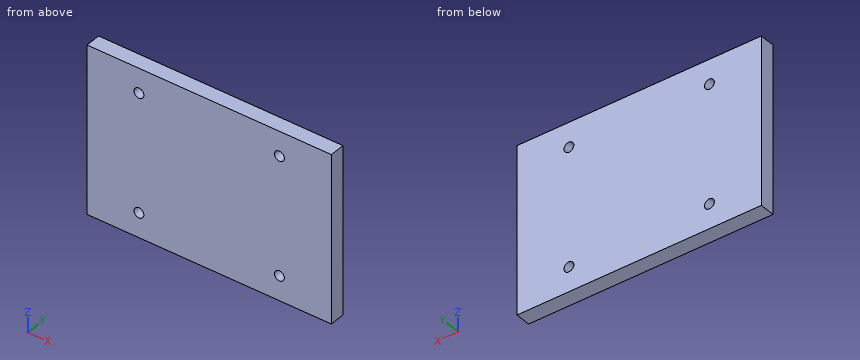
Autodesk Inventor part; units mm, degrees
ref_plane "YZ Plane" through (0, 0, 0) normal (1, 0, 0) x (0, 1, 0)
ref_plane "XZ Plane" through (0, 0, 0) normal (0, 1, 0) x (-1, 0, 0)
ref_plane "XY Plane" through (0, 0, 0) normal (0, 0, 1) x (1, 0, 0)
sketch "Boceto1" plane through (0, 0, 0) normal (0, 1, 0) x (-1, 0, 0)
  line L0 (0, 0) -> (-80, 0)
  line L1 (-80, 0) -> (-80, -54.52)
  line L2 (-80, -54.52) -> (0, -54.52)
  line L3 (0, -54.52) -> (0, 0)
  line L4 (-80, -54.52) -> (-63, -54.52) construction
  line L5 (-63, -54.52) -> (-63, -46.52) construction
  line L6 (-63, 0) -> (-63, -8) construction
  line L7 (0, -54.52) -> (-17, -54.52) construction
  line L8 (-17, -54.52) -> (-17, -46.52) construction
  line L9 (-17, 0) -> (-17, -8) construction
  dimension "d0" = 80
  dimension "d1" = 54.52
  dimension "d2" = 17
  dimension "d3" = 8
  dimension "d6" = 8
  dimension "d7" = 17
extrude "Extrusión1" add sketch "Boceto1" along normal blind 5
hole "Agujero2" at (63, 0, -46.52) direction (0, 1, 0) diameter 3.242 end through all
hole "Agujero3" at (17, 0, -46.52) at (63, 0, -8) at (17, 0, -8) direction (0, 1, 0) diameter 3.242 end through all
equation "\"Radio_pliegue\" = Grosor"
equation "\"Anchura_desahogo_plegado\" = Grosor"
equation "\"Profundidad_desahogo_plegado\" = 0.5 * Grosor"
equation "\"Tamaño_destalonado\" = 4 * Grosor"
equation "\"Remanente_mínimo\" = 2 * Grosor"
equation "\"Radiodetransición\" = Radio_pliegue"
equation "\"Tamaño_de_radio_de_Jacobi\" = Radio_pliegue"
equation "\"TamañoSeparación\" = Grosor"
properties part number "practica 13.2"
Could you check a few things on this model? Use its own coordinates, in mm. Give positions to 0.01 mm unless a question says otherwise; leave off trailing zeros. Order: outer loops, then holes, each group sorted by start corner. A loop starts at its lowest first (then second) coordinate and runs counter-clockwise, first axis right, second up.
1. Suppose I cut it at B-B (z = -46.52). Write out the boundary of the cut face in (x, y).
Answers below:
outline: (0, 0) - (15.38, 0) - (15.38, 5) - (0, 5) - close; (18.62, 0) - (61.38, 0) - (61.38, 5) - (18.62, 5) - close; (64.62, 0) - (80, 0) - (80, 5) - (64.62, 5) - close
2. For pin 1 (3.5 mm diameter, centred on x = 17, z = -8, fed in from -Y), with a flat end and sliding along its axis, tell me the tip position at first contact or that it passes through.
Answers below:
pin 1: stops at y = 0
3. Suppose I cut it at A-A (x = 17). Write out the boundary of the cut face in (y, z), plus the area to 3 significant figures.
Answers below:
outline: (0, -54.52) - (5, -54.52) - (5, -48.14) - (0, -48.14) - close; (0, -44.9) - (5, -44.9) - (5, -9.62) - (0, -9.62) - close; (0, -6.38) - (5, -6.38) - (5, 0) - (0, 0) - close
area: 240 mm2
4. I need wall thicknesses on L1, parallel to Z at x = 17, y = 2; L2, parallel to X at y = 2.6, z = -46.52; L3, parallel to Z at x = 62.5, y = 3.95. Which ranges of each line are inside material? Lowest first, please.
Answers below:
L1: z = -54.52 to -48.14, -44.9 to -9.62, -6.38 to 0
L2: x = 0 to 15.38, 18.62 to 61.38, 64.62 to 80
L3: z = -54.52 to -48.06, -44.98 to -9.54, -6.46 to 0
